Source: CAD feature listing. Evaluate the final solid. Frame: model axes, mm. A direction names the side the tool comes from. Give positions to 0.01 mm unless a question says otherwise; leave off trailing zeros. Loops run counter-clockwise (first coordinate to the right, second up) from the corner with the lowest first, then second, coordinate; pieces in that order, holes last. Notation, with made-up numbers: M 85.25,80 L 117.25,80 A22 ccw 117.25,102 Z; hole C 28.5,-24.5 d7. An arc over 180 degrees is marked long. Write item = value, one per line.
Autodesk Inventor part; units mm, degrees
ref_plane "Work Plane1" through (5, 0, 0) normal (0, 0, 1) x (1, 0, 0)
ref_plane "YZ Plane" through (0, 0, 0) normal (1, 0, 0) x (0, 1, 0)
ref_plane "XZ Plane" through (0, 0, 0) normal (0, 1, 0) x (-1, 0, 0)
sketch "Sketch1" plane through (0, 0, 0) normal (0, 0, 1) x (1, 0, 0)
  line L0 (0, 0) -> (6.1667, 0)
  line L1 (10, 1.4434) -> (10, 2.5)
  line L2 (10, 2.5) -> (0, 2.5)
  line L3 (10, 1.4434) -> (7, 1.4434)
  line L4 (7, 1.4434) -> (6.1667, 0)
  line L5 (0, -0.5) -> (0, 3)
  line L6 (0, 2.5) -> (0, 0)
  dimension "d0" = 3
  dimension "d1" = 60
  dimension "d2" = 5
  dimension "d3" = 2.8868
  dimension "d5" = 10
revolve "Body" add sketch "Sketch1" angle 360 about axis through (0, 0, 0) along (1, 0, 0)
sketch "Sketch2" plane through (10, 0, 0) normal (1, 0, 0) x (0, 1, 0)
  circle A0 centre (0, 0) radius 1.4434
  line L0 (-0.7217, 1.25) -> (0.7217, 1.25)
  line L1 (0.7217, 1.25) -> (1.4434, 0)
  line L2 (1.4434, 0) -> (0.7217, -1.25)
  line L3 (0.7217, -1.25) -> (-0.7217, -1.25)
  line L4 (-0.7217, -1.25) -> (-1.4434, 0)
  line L5 (-1.4434, 0) -> (-0.7217, 1.25)
  point P0 (0, 0)
  point P1 (0, 0)
extrude "Slot" add sketch "Sketch2" against normal up to next contours L1 A0 | A0 L2 | L0 A0 | A0 L3 | L5 A0 | A0 L4
thread "Thread"
chamfer "Chamfer1" distance 2.5 angle 45 1 edges at (0, -2.5, 0) measured on face at (6.6667, 2.4919, -0.2012)
chamfer "Chamfer2" distance 0.4908 angle 45 1 edges at (10, -2.5, 0) measured on face at (7.4998, 2.4676, -0.401)
ref_plane "Work Plane1" through (5, 0, 0) normal (0, 0, 1) x (1, 0, 0)
equation "\"d0\" = INTI"
equation "\"d2\" = NND"
equation "\"d3\" = 1.1547 * SW"
equation "\"d5\" = NLG"
equation "\"d12\" = NLG"
equation "\"d9\" = FAWI"
equation "\"d10\" = -0.5 * GD1 + 0.5 * NND"
equation "\"d11\" = FAWI"
equation "\"d35\" = -0.5 * GD1 + 0.5 * NND"
equation "\"NND\" = 5"
equation "\"NLG\" = 10"
equation "\"INTI\" = 3"
equation "\"FAWI\" = 45deg"
equation "\"SW\" = 2.5"
equation "\"GD1\" = THREADDIA - 1.2269 * PTC"
equation "\"FAWI1\" = 45deg"
equation "\"SPD\" = 0.00001"
equation "\"GUL\" = 0.61345 * PTC"
equation "\"TOA\" = 30deg"
equation "\"THREADDIA\" = 5"
equation "\"PTC\" = 0.8"
equation "\"GAL\" = 0.61345 * PTC"
equation "\"E0\" = 1.155 * SW"
properties part number "DIN 914 - M5 x 10" material "Steel, Mild"
1. Cut plane B-B, the plane x = 5.25. Return the cut outline in (y, z).
Derived:
outline = C 0,0 d5
2. Reachability of faces 1 (the flat face through (8.466, 1.088, -0.616)), 2 (the cylindrical face through (5.96, -0.54, 2.44)) from +Z, -Z, +X, -X, +Y, -Y: full face, straight path, thin tool, end or side. Return the list, or none.
Derived:
face_1 = +X
face_2 = +X, -X
3. Cut plane A-A, the plane x = 7.25. Return the cut outline in (y, z), then the cut area to 3 significant figures.
Derived:
outline = C 0,0 d5; hole M -1.44,0 L -0.72,-1.25 L 0.72,-1.25 L 1.44,0 L 0.72,1.25 L -0.72,1.25 Z
area = 14.2 mm²
4. Pull-direction query (Y, two-part tool) for faces 3 (the conical face through (1, 0, -1)), 4 (the flat face through (8, 0, 1.25)); classes: +Y half, -Y half, draft (parallel to the pull), parting line (faces both ways), or undercut.
Derived:
face_3 = parting line
face_4 = undercut
5. Cut plane C-C, the plane x = 0.5. Return the cut outline in (y, z), then the cut area to 3 significant figures.
Derived:
outline = C 0,0 d1
area = 0.785 mm²
6. First-contact query: pin 1 Ø3 at (x, z) = (8, 1) entering from +Y; pin 2 Ø1.5 at (y, z) = (-0.5, -1) entering from -X; pin 3 Ø1.5 at (y, z) = (-1.5, -1) entering from -X. Flat tips, straight axial feed; report the tip coordinate or a pass-through.
Derived:
pin_1 = 2.5
pin_2 = 0.37
pin_3 = 1.05
7. Material intervals for probe 1 along Z at (x, y) = (8.75, 0.5); probe 2 along Y at (x, z) = (8.5, -0.25); probe 3 along Z at (x, y) = (5.25, -1), sorted ascending. Write a range as from..to.
Derived:
probe_1 = -2.45..-1.25, 1.25..2.45
probe_2 = -2.49..-1.3, 1.3..2.49
probe_3 = -2.29..2.29
